Build history of the part. All positions in model axes, mm. A direction names the side the tool comes from. Round coordinates to 2 decimals unless told otherwise and drop trailing zeros. Write each loop counter-clockwise with the first axis right and the second up, starting at its lowest first coordinate (ties: lowest second). Pieces come first, ordered by that corner, then holes. Notation, with made-up numbers: (34, -27) - (71, -27) arc R21 ccw to (71, -13) - close; hole circle Ø3 at (54.5, -30.5). An arc over 180 degrees is marked (long way). Answer as a JSON object with one key per item and string values. Group by question number.
Item 1: Two-plate mould, pull along X, no slides. Class faces 1 (the flat face through (0, 6, 8)), 2 (the flat face through (-1, 6, 27)), 3 (the cylindrical face through (5.948, 6.388, 18.017)): +X half, -X half, draft (parallel to the pull), parting line (faces both ways), or undercut.
Item 2: Slice it at A-A, the plane z = 60.2. List the corners of the cut face in (x, y).
Item 3: Which spindle directions (+Z, -Z, +X, -X, +Y, -Y) get a long thin tool onto all of the face, cutting with end or side? Do faces 4 (the flat face through (-1, 6, 17)), 5 (the flat face through (0, 7, 59)), 6 (the flat face through (5, 12.6, 62)). Say none if no direction does.
Item 4: Flat gauge pins, fed straight in: pin 1 (2 mm diameter, centred on x = 5, z = 13, fed in from +Y); pin 2 (4 mm diameter, centred on y = 7.5, z = 8, fed in from -X); pin 3 (0.8 mm diameter, centred on x = -1, y = 6, fed in from -Z). Where does each tip first touch, or does it go through?
Item 5: Slice it at B-B, the plane y = 3.75. List the corners of the cut face in (x, z), then the cut area to 3 significant figures.
Item 6: Probe line 1 (X direction, y = 8.5, z = 5); line 2 (Z direction, x = 9.5, y = 1.5); line 3 (Z direction, x = 6, y = 9.25). List the from-to ranges inside material, lowest first. Write a range as from..to.
Item 7: Slice it at D-D, the plane z = 20. List the corners of the cut face in (x, y).
Item 8: Slice it at C-C, the plane x = 1.25. List the corners of the cut face in (y, z).
from build123d import *

# Parameters (mm, degrees)
ESQUISSE1_W             = 12.6
ESQUISSE1_H             = 12.6
BOSS_EXTRU_1_DEPTH      = 80.2
ESQUISSE2_R             = 1.5
ESQUISSE2_R_2           = 2
ENL_V_MAT_EXTRU_1_DEPTH = 13.6
ESQUISSE3_R             = 5.35
ENL_V_MAT_EXTRU_4_DEPTH = 13.6
ESQUISSE4_W             = 12.6
ESQUISSE4_H             = 14
BOSS_EXTRU_2_DEPTH      = 1.5
ESQUISSE5_W             = 10
ESQUISSE5_H             = 12.6
BOSS_EXTRU_3_DEPTH      = 1.5


with BuildPart() as part:
    # Esquisse1 → Boss.-Extru.1 (new body)
    with BuildSketch(Plane.XY):
        with Locations((6.3, 6.3)):
            Rectangle(ESQUISSE1_W, ESQUISSE1_H)
    extrude(amount=BOSS_EXTRU_1_DEPTH)

    # Esquisse2 → Enlèv. mat.-Extru.1 (cut, through all)
    with BuildSketch(Plane(origin=(0, 12.6, 0), x_dir=(1, 0, 0), z_dir=(0, 1, 0))):
        with Locations((6.208458314, -75.2)):
            Circle(ESQUISSE2_R)
        with Locations((6.208458314, -60.2)):
            Circle(ESQUISSE2_R)
        with Locations((6.208458314, -20)):
            Circle(ESQUISSE2_R_2)
        with Locations((6.208458314, -5)):
            Circle(ESQUISSE2_R_2)
    extrude(amount=-ENL_V_MAT_EXTRU_1_DEPTH, mode=Mode.SUBTRACT)

    # Esquisse3 → Enlèv. mat.-Extru.4 (cut, through all)
    with BuildSketch(Plane(origin=(12.6, 0, 0), x_dir=(0, 0, -1), z_dir=(1, 0, 0))):
        with Locations((-33.35, 6.3)):
            Circle(ESQUISSE3_R)
        with Locations((-40.75, 6.3)):
            Circle(ESQUISSE3_R)
    extrude(amount=-ENL_V_MAT_EXTRU_4_DEPTH, mode=Mode.SUBTRACT)

    # Esquisse4 → Boss.-Extru.2 (add)
    with BuildSketch(Plane(origin=(0, 12.6, 0), x_dir=(1, 0, 0), z_dir=(0, 1, 0))):
        with Locations((6.3, -36.5)):
            Rectangle(ESQUISSE4_W, ESQUISSE4_H)
    extrude(amount=BOSS_EXTRU_2_DEPTH)

    # Esquisse5 → Boss.-Extru.3 (add)
    with BuildSketch(Plane.ZY):
        with Locations((22, 6.3)):
            Rectangle(ESQUISSE5_W, ESQUISSE5_H)
    extrude(amount=BOSS_EXTRU_3_DEPTH)


solid = part.part
Geometry says:
{
 "1": {"face 1": "-X half", "face 2": "draft", "face 3": "undercut"},
 "2": {"outline": "(0, 0) - (4.71, 0) - (4.71, 12.6) - (0, 12.6) - close; (7.71, 0) - (12.6, 0) - (12.6, 12.6) - (7.71, 12.6) - close"},
 "3": {"face 4": "-Z, -X, +Y, -Y", "face 5": "+Z, -X, +Y, -Y", "face 6": "+Z, +X, -X, +Y"},
 "4": {"pin 1": "stops at y = 12.6", "pin 2": "stops at x = 0", "pin 3": "stops at z = 17"},
 "5": {"outline": "(-1.5, 17) - (0, 17) - (0, 0) - (12.6, 0) - (12.6, 28.65) - (0, 28.65) - (0, 27) - (-1.5, 27) - close; (0, 45.45) - (12.6, 45.45) - (12.6, 80.2) - (0, 80.2) - close; hole circle Ø4 at (6.21, 5); hole circle Ø4 at (6.21, 20); hole circle Ø3 at (6.21, 60.2); hole circle Ø3 at (6.21, 75.2)", "area": "774 mm^2"},
 "6": {"line 1": "x = 0..4.21, 8.21..12.6", "line 2": "z = 0..30.99, 35.71..38.39, 43.11..80.2", "line 3": "z = 0..3.01, 6.99..18.01, 21.99..28.89, 45.21..58.71, 61.69..73.71, 76.69..80.2"},
 "7": {"outline": "(-1.5, 0) - (4.21, 0) - (4.21, 12.6) - (-1.5, 12.6) - close; (8.21, 0) - (12.6, 0) - (12.6, 12.6) - (8.21, 12.6) - close"},
 "8": {"outline": "(0, 0) - (12.6, 0) - (12.6, 29.5) - (14.1, 29.5) - (14.1, 43.5) - (12.6, 43.5) - (12.6, 80.2) - (0, 80.2) - close; hole (2.44, 37.05) arc R5.35 ccw (long way) to (10.16, 37.05) arc R5.35 ccw (long way) to start"}
}
